Could you check a few things on this model? Use its own coordinates, in mm. Coordinates: 2 decimals unless noted, no trailing zeros. Write each loop counter-clockwise with the first axis right and the second up, starting at its lowest first coordinate (ties: lowest second). Pieces come first, ordered by that corner, then holes. Notation, with made-up numbers: (-26.5, 18.5) - (19.5, 18.5) arc R20 ccw to (19.5, 29.5) - close; hole circle Ø7 at (-12.75, 9.25). An arc over 180 degrees is marked (long way). Answer as a JSON object with one key per item and string values. Group by question number.
1) If we section it at A-A (x = 325): Write out the boundary of the cut face in (y, z), plus the area to 3 significant figures.
2) Will this pin go through, and if not, where does the flat tip stop? pin 1 Ø23.5 at (x, y) = (551.74, -45.78) entering from +Z.
3) Please list where these lines run through material, in increasing order: line 1 along Y through (x, z) = (321, 3.5); line 2 along X through (y, z) = (-645, 10.5); line 3 along Y through (x, z) = (645, 5.75).
4) If we section it at C-C (z = 11): Write out the boundary of the cut face in (x, y), plus the area to 3 significant figures.
5) If we section it at B-B (y = -325): Write out the boundary of the cut face in (x, z), plus the area to 3 significant figures.
6) We'd pull the mould along Y, two halves only. Please class faces 1 (the flat face through (0, -330, 10)), 2 (the flat face through (320, -650, 10)), 3 (the cylindrical face through (473.98, -95.05, 10.14)): released by +Y, released by -Y, zero draft, split by the parting line, or undercut.
```python
from build123d import *

# Parameters (mm, degrees)
F0_W       = 650
F0_H       = 650
F1_DEPTH   = 20
F2_R       = 50
F3_DEPTH   = 25
F4_R       = 26.673415
F9_DEPTH   = 25
F5_R       = 21.925408
F10_DEPTH  = 25
F6_R       = 16.384006
F11_DEPTH  = 25
F7_R       = 14.701481
F12_DEPTH  = 25
F8_R       = 9.686961
F13_DEPTH  = 25
F11_FACE_R = 16.384006
F14_DEPTH  = 50
F15_R      = 3
F16_DEPTH  = 25


with BuildPart() as f1:
    # F0 (on Top) → F1 (new body)
    with BuildSketch(Plane.XY):
        with Locations((325, -325)):
            Rectangle(F0_W, F0_H)
    extrude(amount=F1_DEPTH)

    # F2 (on face) → F3 (cut)
    with BuildSketch(Plane.XY.offset(20)):
        with Locations((325, -325)):
            Circle(F2_R)
    extrude(amount=-F3_DEPTH, mode=Mode.SUBTRACT)

    # F4 (on face) → F9 (cut)
    with BuildSketch(Plane.XY.offset(20)):
        with Locations((381.598979, -227.318332)):
            Circle(F4_R)
    extrude(amount=-F9_DEPTH, mode=Mode.SUBTRACT)

    # F5 (on face) → F10 (cut)
    with BuildSketch(Plane.XY.offset(20)):
        with Locations((437.728018, -156.280026)):
            Circle(F5_R)
    extrude(amount=-F10_DEPTH, mode=Mode.SUBTRACT)

    # F6 (on face) → F11 (join)
    with BuildSketch(Plane.XY.offset(20)):
        with Locations((490.348995, -95.765911)):
            Circle(F6_R)
    extrude(amount=F11_DEPTH)

    # F7 (on face) → F12 (cut)
    with BuildSketch(Plane.XY.offset(20)):
        with Locations((551.74011, -45.775995)):
            Circle(F7_R)
    extrude(amount=-F12_DEPTH, mode=Mode.SUBTRACT)

    # F8 (on face) → F13 (cut)
    with BuildSketch(Plane.XY.offset(20)):
        with Locations((588.574767, -15.080438)):
            Circle(F8_R)
    extrude(amount=-F13_DEPTH, mode=Mode.SUBTRACT)

    # F11_face (on face) → F14 (cut)
    with BuildSketch(Plane(origin=(490.348995, -95.765911, 45), x_dir=(1, 0, 0), z_dir=(0, 0, 1))):
        Circle(F11_FACE_R)
    extrude(amount=-F14_DEPTH, mode=Mode.SUBTRACT)

    # F15 (on face) → F16 (cut)
    with BuildSketch(Plane.XY.offset(20)):
        with Locations((645, -645)):
            Circle(F15_R)
    extrude(amount=-F16_DEPTH, mode=Mode.SUBTRACT)


solid = f1.part
```
Here are the results:
{
 "1": {"outline": "(-650, 0) - (-375, 0) - (-375, 20) - (-650, 20) - close; (-275, 0) - (0, 0) - (0, 20) - (-275, 20) - close", "area": "11,000 mm²"},
 "2": {"pin 1": "passes through"},
 "3": {"line 1": "y = -650 to -374.84, -275.16 to 0", "line 2": "x = 0 to 642, 648 to 650", "line 3": "y = -650 to -648, -642 to 0"},
 "4": {"outline": "(0, -650) - (650, -650) - (650, 0) - (0, 0) - close; hole circle Ø100 at (325, -325); hole circle Ø53.35 at (381.6, -227.32); hole circle Ø43.85 at (437.73, -156.28); hole circle Ø32.77 at (490.35, -95.77); hole circle Ø29.4 at (551.74, -45.78); hole circle Ø19.37 at (588.57, -15.08); hole circle Ø6 at (645, -645)", "area": "409,000 mm²"},
 "5": {"outline": "(0, 0) - (275, 0) - (275, 20) - (0, 20) - close; (375, 0) - (650, 0) - (650, 20) - (375, 20) - close", "area": "11,000 mm²"},
 "6": {"face 1": "zero draft", "face 2": "released by -Y", "face 3": "undercut"}
}
